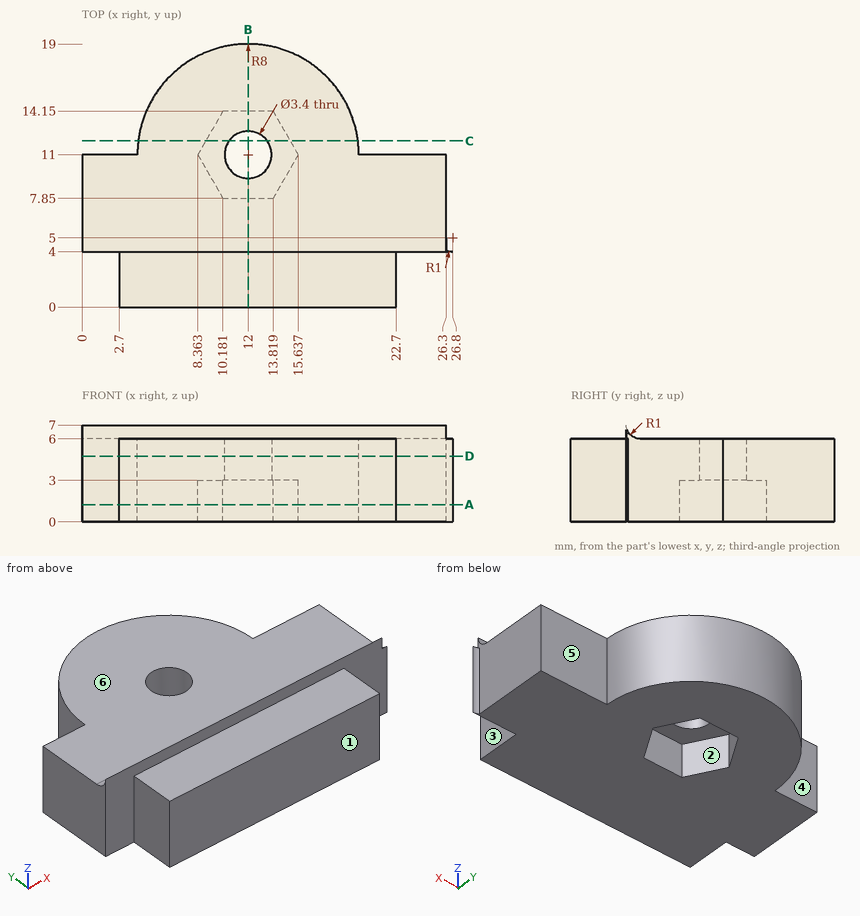
Drawing for the job (mm, zero at the part's lowest x, y, z). A direction names the side the tool comes from. Round coordinates to 2 decimals unless told otherwise and drop trailing zeros. Loops run counter-clockwise (first coordinate to the right, second up) from the corner with the lowest first, then second, coordinate; pieces in that order, holes last. Notation, with made-up numbers: (-28.5, 30) -> (-11.5, 30) arc R19 cw to (-11.5, 59) -> close; hole circle Ø5 at (27, 47.5). An arc over 180 degrees is marked (long way). Answer as CSV lines item,"result". Start each with the question number.
1) Probe line 1 along Y through (x, z) = (12, 4.75); line 2 along Y through (x, z) = (21.5, 4.75); line 3 along Z through (x, y) = (3, 5.5). List the from-to ranges inside material, lowest first.
2) Mould opens along X. For the marked faces 1, 2 and 3 say: +X half, -X half, draft (parallel to the pull), parting line (faces both ways), or undercut.
3) Slice it at A-A (z = 1.25). List the corners of the cut face in (x, y).
4) Tool access for the marked faces 4, 5 and 6: list every direction of +Z, -Z, +X, -X, +Y, -Y with a clear straight run to the whole face (end or side of a thin tool).
5) Slice it at B-B (x = 12). List the corners of the cut face in (y, z).
6) Slice it at D-D (z = 4.75). List the corners of the cut face in (x, y).
7) Slice it at C-C (y = 12). List the corners of the cut face in (x, z) (1 decimal).
8) Pin check, flat tips, straight feed: P1, Ø3, axis at y = 2, z = 1.5, coming from the -X side; P2, Ø1.2, axis at x = 2, z = 1.5, coming from the +Y side; P3, Ø4, axis at x = 16, y = 13, coming from the +Z side. Stop position of each tip, or through.
Filled in:
1,line 1,"y = 0 to 9.3, 12.7 to 19"
1,line 2,"y = 0 to 11"
1,line 3,"z = 0 to 6"
2,face 1,"draft"
2,face 2,"undercut"
2,face 3,"+X half"
3,outline,"(0, 4) -> (2.7, 4) -> (2.7, 0) -> (22.7, 0) -> (22.7, 4) -> (26.8, 4) arc R1 cw to (26.3, 4.13) -> (26.3, 11) -> (20, 11) arc R8 ccw to (4, 11) -> (0, 11) -> close; hole (8.36, 11) -> (10.18, 7.85) -> (13.82, 7.85) -> (15.64, 11) -> (13.82, 14.15) -> (10.18, 14.15) -> close"
4,face 4,"+Z, -Z, -X, +Y"
4,face 5,"+Z, -Z, +X, +Y"
4,face 6,"+Z, +X, -X, +Y"
5,outline,"(0, 0) -> (7.85, 0) -> (7.85, 3) -> (9.3, 3) -> (9.3, 6) -> (5, 6) arc R1 cw to (4, 7) -> (4, 6) -> (0, 6) -> close; (12.7, 3) -> (14.15, 3) -> (14.15, 0) -> (19, 0) -> (19, 6) -> (12.7, 6) -> close"
6,outline,"(0, 4) -> (2.7, 4) -> (2.7, 0) -> (22.7, 0) -> (22.7, 4) -> (26.8, 4) arc R1 cw to (26.3, 4.13) -> (26.3, 11) -> (20, 11) arc R8 ccw to (4, 11) -> (0, 11) -> close; hole circle Ø3.4 at (12, 11)"
7,outline,"(4.1, 0) -> (8.9, 0) -> (8.9, 3) -> (10.6, 3) -> (10.6, 6) -> (4.1, 6) -> close; (13.4, 3) -> (15.1, 3) -> (15.1, 0) -> (19.9, 0) -> (19.9, 6) -> (13.4, 6) -> close"
8,P1,"stops at x = 2.7"
8,P2,"stops at y = 11"
8,P3,"stops at z = 6"
